Part model, mm, in its own coordinate system. A direction names the side the tool comes from. Coordinates: 2 decimals unless noted, no trailing zeros. Write each loop counter-clockwise with the first axis right and the second up, starting at its lowest first coordinate (ties: lowest second). Pieces come first, ordered by that corner, then holes. Notation, with made-up numbers: (21.5, -23.75) -> (44.5, -23.75) arc R21 ccw to (44.5, 1.25) -> close; hole circle Ø1 at (55, -1). An arc over 180 degrees is marked (long way). Write item = value, one per line.
from build123d import *

# Parameters (mm, degrees)
SKETCH1_R           = 7.5
SKETCH1_R_2         = 4.2
BOSS_EXTRUDE1_DEPTH = 47
SKETCH2_R           = 11.2
CUT_EXTRUDE1_DEPTH  = 7
SKETCH3_R           = 2.25
SKETCH3_R_2         = 12
CUT_EXTRUDE2_DEPTH  = 15
CUT_EXTRUDE3_DEPTH  = 48
CUT_EXTRUDE4_DEPTH  = 20
SKETCH7_R           = 2.6
CUT_EXTRUDE5_DEPTH  = 10
SKETCH8_R           = 2.6
CUT_EXTRUDE6_DEPTH  = 8
CHAMFER1_SIZE       = 1
SKETCH9_R           = 2.6
CUT_EXTRUDE7_DEPTH  = 10
CHAMFER2_SIZE       = 1


with BuildPart() as part:
    # Sketch1 → Boss-Extrude1 (new body)
    with BuildSketch(Plane.XY):
        Polygon((-30, -25), (-30, 22), (22, 22), (52, 8), (52, -25), align=None)
        Circle(SKETCH1_R, mode=Mode.SUBTRACT)
        with Locations((40, 0)):
            Circle(SKETCH1_R_2, mode=Mode.SUBTRACT)
    extrude(amount=BOSS_EXTRUDE1_DEPTH)

    # Sketch2 → Cut-Extrude1 (cut)
    with BuildSketch(Plane.XY.offset(47)):
        Circle(SKETCH2_R)
    extrude(amount=-CUT_EXTRUDE1_DEPTH, mode=Mode.SUBTRACT)

    # Sketch3 → Cut-Extrude2 (cut)
    with BuildSketch(Plane(origin=(0, 0, 0), x_dir=(-1, 0, 0), z_dir=(0, 0, -1))):
        with Locations((-15.5, 15.5)):
            Circle(SKETCH3_R)
        with Locations((-15.5, -15.5)):
            Circle(SKETCH3_R)
        with Locations((15.5, -15.5)):
            Circle(SKETCH3_R)
        with Locations((15.5, 15.5)):
            Circle(SKETCH3_R)
        Circle(SKETCH3_R_2)
    extrude(amount=-CUT_EXTRUDE2_DEPTH, mode=Mode.SUBTRACT)

    # Sketch4 → Cut-Extrude3 (cut, through all)
    with BuildSketch(Plane(origin=(0, 22, 0), x_dir=(1, 0, 0), z_dir=(0, 1, 0))):
        with BuildLine():
            Line((-19, -7), (41, -7))
            ThreePointArc((41, -7), (44.535533906, -8.464466094), (46, -12))
            Line((46, -12), (46, -32))
            ThreePointArc((46, -32), (44.535533906, -35.535533906), (41, -37))
            Line((41, -37), (-19, -37))
            ThreePointArc((-19, -37), (-22.535533906, -35.535533906), (-24, -32))
            Line((-24, -32), (-24, -12))
            ThreePointArc((-24, -12), (-22.535533906, -8.464466094), (-19, -7))
        make_face()
    extrude(amount=-CUT_EXTRUDE3_DEPTH, mode=Mode.SUBTRACT)

    # Sketch6 → Cut-Extrude4 (cut)
    with BuildSketch(Plane.XY.offset(47)):
        with BuildLine():
            Line((-19.5, -12), (-19.5, -18))
            ThreePointArc((-19.5, -18), (-15.5, -22), (-11.5, -18))
            Line((-11.5, -18), (-11.5, -12))
            ThreePointArc((-11.5, -12), (-15.5, -8), (-19.5, -12))
        make_face()
        with BuildLine():
            Line((11.5, -12), (11.5, -18))
            ThreePointArc((11.5, -18), (15.5, -22), (19.5, -18))
            Line((19.5, -18), (19.5, -12))
            ThreePointArc((19.5, -12), (15.5, -8), (11.5, -12))
        make_face()
    extrude(amount=-CUT_EXTRUDE4_DEPTH, mode=Mode.SUBTRACT)

    # Sketch7 → Cut-Extrude5 (cut)
    with BuildSketch(Plane(origin=(52, 0, 0), x_dir=(0, 0, -1), z_dir=(1, 0, 0))):
        with Locations(Location((-42, 0, 0), (0, 0, 90))):  # turned: the seam where the file's is
            Circle(SKETCH7_R)
    extrude(amount=-CUT_EXTRUDE5_DEPTH, mode=Mode.SUBTRACT)

    # Sketch8 → Cut-Extrude6 (cut)
    with BuildSketch(Plane.XZ.offset(25)):
        with Locations((-25, 42)):
            Circle(SKETCH8_R)
        with Locations((-25, 5)):
            Circle(SKETCH8_R)
        with Locations((47, 5)):
            Circle(SKETCH8_R)
        with Locations((47, 42)):
            Circle(SKETCH8_R)
    extrude(amount=-CUT_EXTRUDE6_DEPTH, mode=Mode.SUBTRACT)

    # Chamfer1
    chamfer1_edges = [part.edges().sort_by_distance(p)[0] for p in [
        (-27.6, -25, 42),
        (-27.6, -25, 5),
        (44.4, -25, 5),
        (44.4, -25, 42),
    ]]
    chamfer(chamfer1_edges, length=CHAMFER1_SIZE)

    # Sketch9 → Cut-Extrude7 (cut)
    with BuildSketch(Plane.ZY.offset(30)):
        with Locations((41, 12)):
            Circle(SKETCH9_R)
        with Locations((21, 12)):
            Circle(SKETCH9_R)
    extrude(amount=-CUT_EXTRUDE7_DEPTH, mode=Mode.SUBTRACT)

    # Chamfer2
    chamfer2_edges = [part.edges().sort_by_distance(p)[0] for p in [
        (52, -2.6, 42),
    ]]
    chamfer(chamfer2_edges, length=CHAMFER2_SIZE)


solid = part.part
Q1. Mould opens along X. For faces 5 (the face through (-25.07, 10.418, 38.937)), 6 (the face through (-20, 12, 41)), 7 (the face through (15.6, -8, 42.1)) say: released by +X, released by -X, zero draft, split by the parting line, or undercut.
Model answer:
face_5 = zero draft
face_6 = released by -X
face_7 = undercut
Q2. Pin check, flat tips, straight feed: pin 1 (4 mm diameter, centred on x = 47, z = 5, fed in from +Y); pin 2 (4.5 mm diameter, centred on x = 47, z = 42, fed in from -Y); pin 3 (5 mm diameter, centred on x = 15.5, y = -15.5, fed in from +Z). Stop position of each tip, or through.
Model answer:
pin_1 = 11.27
pin_2 = -17
pin_3 = 7
Q3. Probe line 1 (Z direction, x = -25, y = -20.25); line 2 (Y direction, x = -26.75, z = 41); line 3 (X direction, y = 15, z = 4). List the from-to ranges inside material, lowest first. Write a range as from..to.
Model answer:
line_1 = 0..2.4, 7.6..39.4, 44.6..47
line_2 = -17..9.4, 14.6..22
line_3 = -30..-17.69, -13.31..13.31, 17.69..37
Q4. Saw through at D-D on z = 31. Give the cut face in (x, y), and give its area (3 significant figures).
Model answer:
outline = (-30, -25) -> (-24, -25) -> (-24, 22) -> (-30, 22) -> close; (46, -25) -> (52, -25) -> (52, 8) -> (46, 10.8) -> close
area = 488 mm²
Q5. Which spindle directions (+Z, -Z, +X, -X, +Y, -Y) get a long thin tool onto all of the face, cutting with end or side? Do faces 1 (the face through (11, -1, 37)), 2 (the face through (11.99, 0.53, 3.45)), 3 (the face through (-15.6, -22, 42.1)), 4 (the face through (44.4, -20.5, 5.1)). Say none if no direction does.
Model answer:
face_1 = +Y, -Y
face_2 = -Z
face_3 = +Z
face_4 = -Y
Q6. Saw through at B-B on x = 40. Give the cut face in (y, z).
Model answer:
outline = (-25, 0) -> (-4.2, 0) -> (-4.2, 7) -> (-25, 7) -> close; (-25, 37) -> (-4.2, 37) -> (-4.2, 47) -> (-25, 47) -> close; (4.2, 0) -> (13.6, 0) -> (13.6, 7) -> (4.2, 7) -> close; (4.2, 37) -> (13.6, 37) -> (13.6, 47) -> (4.2, 47) -> close
Q7. Saw through at A-A on z = 21. Give the cut face in (x, y).
Model answer:
outline = (-30, -25) -> (-24, -25) -> (-24, 9.4) -> (-30, 9.4) -> close; (-30, 14.6) -> (-24, 14.6) -> (-24, 22) -> (-30, 22) -> close; (46, -25) -> (52, -25) -> (52, 8) -> (46, 10.8) -> close
Q8. Saw through at C-C on y = -15.5. Give the cut face in (x, z).
Model answer:
outline = (-30, 0) -> (-17.75, 0) -> (-17.75, 7) -> (-19, 7) arc R5 cw to (-24, 12) -> (-24, 32) arc R5 cw to (-19.5, 36.97) -> (-19.5, 47) -> (-30, 47) -> close; (-13.25, 0) -> (13.25, 0) -> (13.25, 7) -> (-13.25, 7) -> close; (-11.5, 37) -> (11.5, 37) -> (11.5, 47) -> (-11.5, 47) -> close; (17.75, 0) -> (52, 0) -> (52, 47) -> (19.5, 47) -> (19.5, 37) -> (41, 37) arc R5 cw to (46, 32) -> (46, 12) arc R5 cw to (41, 7) -> (17.75, 7) -> close
